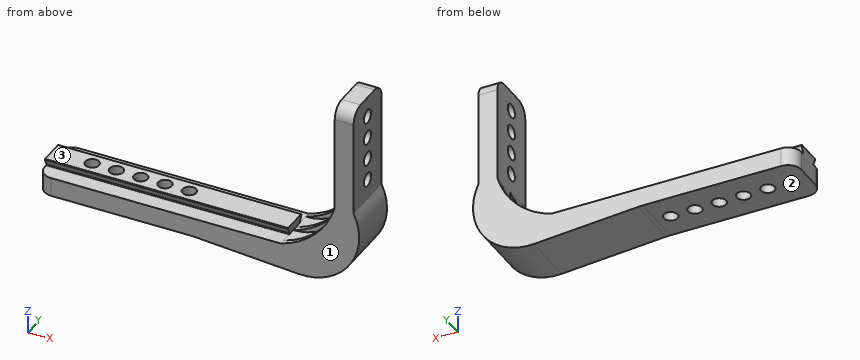
from build123d import *

# Parameters (mm, degrees)
BOSS_EXTRUDE1_DEPTH = 20
BOSS_EXTRUDE2_DEPTH = 90
SKETCH4_R           = 2.55
CUT_EXTRUDE1_DEPTH  = 137.301137193
LPATTERN1_COUNT     = 4
LPATTERN1_PITCH     = 8.3
SKETCH5_R           = 2.55
CUT_EXTRUDE2_DEPTH  = 14
LPATTERN2_COUNT     = 5
LPATTERN2_PITCH     = 9
FILLET2_R           = 5
BOSS_EXTRUDE4_DEPTH = 20
BOSS_EXTRUDE5_DEPTH = 2
LPATTERN3_COUNT     = 3
LPATTERN3_PITCH     = 9
FILLET3_R           = 0.3
FILLET4_R           = 20


with BuildPart() as part:
    # Sketch1 → Boss-Extrude1 (new body)
    with BuildSketch(Plane(origin=(0, 0, 0), x_dir=(1, 0, 0), z_dir=(0, 1, 0))):
        with BuildLine():
            Line((0, 0), (90, 0))
            ThreePointArc((90, 0), (109.091883092, -7.908116908), (117, -27))
            Line((117, -27), (117, -67))
            Line((117, -67), (110, -67))
            Line((110, -67), (110, -27))
            ThreePointArc((110, -27), (104.142135624, -12.857864376), (90, -7))
            Line((90, -7), (0, -7))
            Line((0, -7), (0, 0))
        make_face()
    extrude(amount=BOSS_EXTRUDE1_DEPTH)

    # Sketch2 → Boss-Extrude2 (add)
    with BuildSketch(Plane(origin=(0, 0, 0), x_dir=(0, 0, -1), z_dir=(1, 0, 0))):
        Polygon((-10, 15), (-10, 5), (-7, 6.398922974), (-7, 13.601077026), align=None)
    extrude(amount=BOSS_EXTRUDE2_DEPTH)

    # Sketch4 → Cut-Extrude1 (cut, through all)
    with BuildSketch(Plane(origin=(0, 0, 0), x_dir=(0, 0, -1), z_dir=(1, 0, 0))):
        with Locations(Location((-59.5, 10, 0), (0, 0, 180))):
            Circle(SKETCH4_R)
    cut_extrude1 = extrude(amount=CUT_EXTRUDE1_DEPTH, mode=Mode.SUBTRACT)

    # LPattern1: Cut-Extrude1 ×4
    with Locations(*[(0, 0, -i * LPATTERN1_PITCH) for i in range(1, LPATTERN1_COUNT)]):
        add(cut_extrude1, mode=Mode.SUBTRACT)

    # Sketch5 → Cut-Extrude2 (cut)
    with BuildSketch(Plane.XY):
        with Locations(Location((15, 10, 0), (0, 0, 90))):
            Circle(SKETCH5_R)
    cut_extrude2 = extrude(amount=CUT_EXTRUDE2_DEPTH, mode=Mode.SUBTRACT)

    # LPattern2: Cut-Extrude2 ×5
    with Locations(*[(i * LPATTERN2_PITCH, 0, 0) for i in range(1, LPATTERN2_COUNT)]):
        add(cut_extrude2, mode=Mode.SUBTRACT)

    # Fillet2
    fillet2_edges = [part.edges().sort_by_distance(p)[0] for p in [
        (0, 0, 3.5),
        (113.5, 20, 67),
        (0, 20, 3.5),
        (113.5, 0, 67),
    ]]
    fillet(fillet2_edges, radius=FILLET2_R)

    # Sketch6 → Boss-Extrude4 (add)
    with BuildSketch(Plane(origin=(0, 0, 0), x_dir=(1, 0, 0), z_dir=(0, 1, 0))):
        with BuildLine():
            Line((57.067989457, 0), (96.460545107, 3))
            ThreePointArc((96.460545107, 3), (115.383129249, -6.075834674), (117, -27))
            ThreePointArc((117, -27), (109.091883092, -7.908116908), (90, 0))
            Line((90, 0), (57.067989457, 0))
        make_face()
    extrude(amount=BOSS_EXTRUDE4_DEPTH)

    # Sketch8 → Boss-Extrude5 (add)
    with BuildSketch(Plane(origin=(0, 0, 0), x_dir=(1, 0, 0), z_dir=(0, 1, 0))):
        with BuildLine():
            ThreePointArc((90, -7), (102.578584062, -14.421415938), (110, -27))
            ThreePointArc((110, -27), (104.142135624, -12.857864376), (90, -7))
        make_face()
    boss_extrude5 = extrude(amount=BOSS_EXTRUDE5_DEPTH)

    # LPattern3: Boss-Extrude5 ×3
    with Locations(*[(0, i * LPATTERN3_PITCH, 0) for i in range(1, LPATTERN3_COUNT)]):
        add(boss_extrude5)

    # Fillet3
    fillet3_edges = [part.edges().sort_by_distance(p)[0] for p in [
        (45, 13.601077026, 7),
        (45, 15, 10),
        (45, 5, 10),
        (45, 6.398922974, 7),
    ]]
    fillet(fillet3_edges, radius=FILLET3_R)

    # Fillet4
    # the kernel refuses this fillet: 20 mm, written as the material it adds along each edge
    with BuildSketch(Plane(origin=(57.067989457, 0, 0), x_dir=(0.9971126456779296, 0, -0.07593663035162816), z_dir=(0, 1, 0))) as fillet4_piece_1:
        with BuildLine():
            CenterArc((FILLET4_R * 0.0380232084134, FILLET4_R), FILLET4_R, 265.644959248, 4.355040752)
            Line((-FILLET4_R * 0.0379134219382, FILLET4_R * 0.00288735432207), (0, 0))
            Line((0, 0), (FILLET4_R * 0.0380232084134, 0))
        make_face()
    extrude(amount=20)


solid = part.part
The listing builds one solid part. Answer for the finished solid, in the listing's coordinates (mm). Face numbers are marked on the shaded views. A direction names the side the tool comes from. Coordinates: 2 decimals unless noted, no trailing zeros. Write each loop counter-clockwise with the first axis right and the second up, starting at its lowest first coordinate (ties: lowest second). Pieces come first, ordered by that corner, then holes. Notation, with made-up numbers: (-39, 1) - (-30, 1) arc R13 cw to (-30, 18) - close; hole circle Ø3 at (58.5, -20). An arc over 180 degrees is marked (long way). Return JSON: item names as keys, results as strings.
1. Consider line 1 along Y through (x, z) = (115, 59.5); line 2 along X through (y, z) = (10, 3.25); line 3 along X through (y, z) = (10, 5.75). Determine where each line is inside the solid, lowest interval first.
Final values:
{"line 1": "0 to 7.45, 12.55 to 20", "line 2": "0 to 12.45, 17.55 to 21.45, 26.55 to 30.45, 35.55 to 39.45, 44.55 to 48.45, 53.55 to 113.06", "line 3": "0 to 12.45, 17.55 to 21.45, 26.55 to 30.45, 35.55 to 39.45, 44.55 to 48.45, 53.55 to 115.16"}
2. Each of these flat-tipped pins is pushed along its axis until it touches: pin 1 Ø6 at (x, y) = (87.5, 4.5) entering from -Z; pin 2 Ø6 at (x, y) = (31, 9) entering from -Z; pin 3 Ø7 at (x, y) = (50, 11) entering from +Z; pin 4 Ø4.5 at (y, z) = (10, 51.2) entering from +X. Where does it stop, or does it pass through?
Final values:
{"pin 1": "z = -2.55", "pin 2": "z = 0", "pin 3": "z = 10", "pin 4": "through"}
3. The part is cut by section A-A on x = 15. Determine the outline of the cut face in (y, z).
Final values:
{"outline": "(0, 0) - (7.45, 0) - (7.45, 10) - (5.47, 10) arc R0.3 ccw to (5.2, 9.57) - (6.2, 7.43) arc R0.3 cw to (5.93, 7) - (0, 7) - close; (12.55, 0) - (20, 0) - (20, 7) - (14.07, 7) arc R0.3 cw to (13.8, 7.43) - (14.8, 9.57) arc R0.3 ccw to (14.53, 10) - (12.55, 10) - close"}
4. The part is cut by section D-D on z = 59.5. Determine the outline of the cut face in (x, y), then the cut area to 3 significant figures.
Final values:
{"outline": "(110, 0) - (117, 0) - (117, 7.45) - (110, 7.45) - close; (110, 12.55) - (117, 12.55) - (117, 20) - (110, 20) - close", "area": "104 mm^2"}
5. The part is cut by section C-C on y = 3.5. Determine the outline of the cut face in (x, z), then the cut area to 3 significant figures.
Final values:
{"outline": "(0.23, 0) - (56.31, 0) arc R20 cw to (57.83, -0.06) - (96.46, -3) arc R21 ccw to (117, 27) - (117, 66.77) - (110, 66.77) - (110, 27) arc R20 cw to (90, 7) - (0.23, 7) - close", "area": "1,400 mm^2"}
6. Which of the six approach directions +Z, -Z, +X, -X, +Y, -Y give full straight-line access (tool end or side, diameter ignored) to the marked faces 1, 2 and 3?
Final values:
{"face 1": "+Z, -Z, +X, -X, -Y", "face 2": "-Z, -X, +Y, -Y", "face 3": "+Z, -X, +Y, -Y"}
7. The part is cut by section B-B on z = 51. Determine the outline of the cut face in (x, y).
Final values:
{"outline": "(110, 0) - (117, 0) - (117, 7.46) - (110, 7.46) - close; (110, 12.54) - (117, 12.54) - (117, 20) - (110, 20) - close"}
